Source: CAD feature listing. Evaluate the final solid. Frame: model axes, mm. A direction names the side the tool comes from. Round coordinates to 2 decimals unless told otherwise and drop trailing zeros. Loops run counter-clockwise (first coordinate to the right, second up) from the corner with the lowest first, then second, coordinate; pieces in that order, holes last. Notation, with made-up numbers: (45.5, 18.5) -> (98.5, 18.5) arc R14 ccw to (98.5, 33.5) -> close; hole circle Ø3 at (5.5, 7). An arc over 180 degrees is marked (long way). Write item = value, one per line.
from build123d import *

# Parameters (mm, degrees)
EXTRUDE1_DEPTH = 5.1308
SKETCH2_W      = 5.207
SKETCH2_H      = 2.54
HOLEWZD1_D     = 4.97586
HOLEWZD1_DEPTH = 7.6708
FILLET1_R      = 0.381
FILLET2_R      = 0.508


with BuildPart() as part:
    # Sketch1 → Extrude1 (new body)
    with BuildSketch(Plane(origin=(0, -2.54, 0), x_dir=(-1, 0, 0), z_dir=(0, 1, 0))):
        Polygon((3.204236259, 5.5499), (-3.204236259, 5.5499), (-6.408472518, 0), (-3.204236259, -5.5499), (3.204236259, -5.5499), (6.408472518, 0), align=None)
    extrude(amount=-EXTRUDE1_DEPTH)

    # Sketch2 → Revolve1 (revolve)
    with BuildSketch(Plane(origin=(0, 0, 0), x_dir=(-1, 0, 0), z_dir=(0, 0, -1))):
        with Locations((-2.6035, -1.27)):
            Rectangle(SKETCH2_W, SKETCH2_H)
    revolve(axis=Axis((0, -2.54, 0), (0, 1, 0)))

    # HoleWzd1
    with Locations(Plane(origin=(0, 0, 0), x_dir=(-1, 0, 0), z_dir=(0, 1, 0))):
        with Locations((0, 0)):
            Hole(HOLEWZD1_D / 2, depth=HOLEWZD1_DEPTH)

    # Fillet1
    fillet1_edges = [part.edges().sort_by_distance(p)[0] for p in [
        (4.806354388, -7.6708, 2.77495),
        (-6.408472518, -5.1054, 0),
        (-3.204236259, -5.1054, -5.5499),
        (3.204236259, -5.1054, -5.5499),
        (6.408472518, -5.1054, 0),
        (3.204236259, -5.1054, 5.5499),
        (-3.204236259, -5.1054, 5.5499),
        (4.806354388, -7.6708, -2.77495),
        (0, -7.6708, -5.5499),
        (-4.806354388, -7.6708, -2.77495),
        (-4.806354388, -7.6708, 2.77495),
        (-4.806354388, -2.54, -2.77495),
        (0, -2.54, -5.5499),
        (4.806354388, -2.54, -2.77495),
        (0, -7.6708, 5.5499),
        (4.806354388, -2.54, 2.77495),
        (0, -2.54, 5.5499),
        (-4.806354388, -2.54, 2.77495),
    ]]
    fillet(fillet1_edges, radius=FILLET1_R)

    # Fillet2
    fillet2_edges = [part.edges().sort_by_distance(p)[0] for p in [
        (-5.207, 0, 0),
    ]]
    fillet(fillet2_edges, radius=FILLET2_R)


solid = part.part
1. Contact query for a flat-ended pin moving along its axis: pin 1 Ø0.6 at (x, z) = (2, 4) entering from +Y. Output: stop coordinate, or through.
Evaluation:
pin_1 = 0
2. Section query A-A (y = -6). Return the cut outline in (x, z).
Evaluation:
outline = (-6.3, -0.19) -> (-3.31, -5.36) arc R0.38 ccw to (-2.98, -5.55) -> (2.98, -5.55) arc R0.38 ccw to (3.31, -5.36) -> (6.3, -0.19) arc R0.38 ccw to (6.3, 0.19) -> (3.31, 5.36) arc R0.38 ccw to (2.98, 5.55) -> (-2.98, 5.55) arc R0.38 ccw to (-3.31, 5.36) -> (-6.3, 0.19) arc R0.38 ccw to start; hole circle Ø4.98 at (0, 0)
3. Section query B-B (y = -2.25). Return the cut outline in (x, z), then the cut area to 3 significant figures.
Evaluation:
outline = circle Ø10.41 at (0, 0); hole circle Ø4.98 at (0, 0)
area = 65.7 mm²
4. Set-up query: faces 1 (the face through (-2.8, -2.54, 4.7)), 2 (the face through (2.7, -2.54, -4.7)), 3 (the face through (4.967, -1.51, -1.564)). Return all of +Z, -Z, +X, -X, +Y, -Y with unobstructed straight access to the full face (end or side cutting, diameter ignored); none if empty.
Evaluation:
face_1 = +Z, -X, +Y
face_2 = -Z, +X, +Y
face_3 = +Y
5. Line query: probe 1 along Z at (x, y) = (0, -2); probe 2 along Z at (x, y) = (0, -4.5); probe 3 along X at (y, z) = (-1.25, 0.5). Output: solid intervals per line, ascending. Write a range as from..to.
Evaluation:
probe_1 = -5.21..-2.49, 2.49..5.21
probe_2 = -5.55..-2.49, 2.49..5.55
probe_3 = -5.18..-2.44, 2.44..5.18
